```python
from build123d import *

# Parameters (mm, degrees)
BOSS_EXTRUDE1_DEPTH      = 6.2
SKETCH2_W                = 5.2
SKETCH2_H                = 28
CUT_EXTRUDE1_DEPTH       = 15.5
SKETCH3_R                = 1.45
BOSS_EXTRUDE2_DEPTH      = 1
DOME1_FACE_RADIUS        = 1.45
DOME1_HEIGHT             = 1.45
SKETCH4_W                = 4
SKETCH4_H                = 8.2
BOSS_EXTRUDE3_DEPTH      = 5
SKETCH5_W                = 3
SKETCH5_H                = 3.5
CUT_EXTRUDE2_DEPTH       = 4.8
SKETCH6_W                = 4
SKETCH6_H                = 2
BOSS_EXTRUDE4_DEPTH      = 1.5
BOSS_EXTRUDE4_TAPER      = 15
BOSS_EXTRUDE5_DEPTH      = 3
BOSS_EXTRUDE5_DEPTH_BACK = 3
SKETCH8_R                = 2
CUT_EXTRUDE3_DEPTH       = 1.5
SKETCH9_R                = 2
CUT_EXTRUDE4_DEPTH       = 1.5
SKETCH10_R               = 2
CUT_EXTRUDE5_DEPTH       = 1.5
SKETCH11_W               = 5.2
SKETCH11_H               = 5.2
CUT_EXTRUDE6_DEPTH       = 2.5
CUT_EXTRUDE6_DRAFT       = -15
SKETCH12_W               = 5.2
SKETCH12_H               = 5.2
CUT_EXTRUDE7_DEPTH       = 2.5
CUT_EXTRUDE7_DRAFT       = -15
SKETCH13_W               = 5.2
SKETCH13_H               = 5.2
CUT_EXTRUDE8_DEPTH       = 2.5
CUT_EXTRUDE8_DRAFT       = -15
SKETCH14_W               = 5.2
SKETCH14_H               = 5.2
CUT_EXTRUDE9_DEPTH       = 2.5
CUT_EXTRUDE9_DRAFT       = -15
SKETCH15_W               = 5.2
SKETCH15_H               = 5.2
CUT_EXTRUDE10_DEPTH      = 2.5
CUT_EXTRUDE10_DRAFT      = -15


with BuildPart() as part:
    # Sketch1 → Boss-Extrude1 (new body)
    with BuildSketch(Plane(origin=(0, 0, 0), x_dir=(0, 0, -1), z_dir=(1, 0, 0))):
        Polygon((0, 0), (0, 3.5), (35, 3.5), (35, 2), (33.5, 2), (33.5, 0), (63.5, 0), (63.5, 16.5), (52, 16.5), (47.468461065, 14.386908691), (46.20060628, 17.105832052), (48.919529641, 18.373686838), (48.919529641, 19.8), (53.5, 19.8), (53.5, 35.663086876), (41.594285018, 35.663086876), (37.062746083, 33.549995567), (35.794891298, 36.268918928), (38.513814659, 37.536773714), (38.513814659, 38.963086876), (43.094285018, 38.963086876), (43.094285018, 55.2), (35.394285018, 55.2), (35.394285018, 68.074097914), (25.594285018, 70.7), (25.594285018, 55.2), (-0.105714982, 55.2), (-0.105714982, 70.7), (-8.705714982, 70.7), (-8.705714982, 55.2), (-16.405714982, 55.2), (-16.405714982, 38.963086876), (-11.825244622, 38.963086876), (-11.825244622, 37.536773714), (-9.106321261, 36.268918928), (-10.374176047, 33.549995567), (-14.905714982, 35.663086876), (-26.811429963, 35.663086876), (-26.811429963, 19.8), (-22.230959604, 19.8), (-22.230959604, 18.373686838), (-19.512036243, 17.105832052), (-20.779891028, 14.386908691), (-25.311429963, 16.5), (-26.811429963, 16.5), (-26.811429963, 11.5), (-18, 11.5), (-18, 0), align=None)
    extrude(amount=BOSS_EXTRUDE1_DEPTH)

    # Sketch2 → Cut-Extrude1 (cut)
    with BuildSketch(Plane(origin=(0, 70.7, 0), x_dir=(1, 0, 0), z_dir=(0, 1, 0))):
        with Locations((3.1, 12.744285018)):
            Rectangle(SKETCH2_W, SKETCH2_H)
    extrude(amount=-CUT_EXTRUDE1_DEPTH, mode=Mode.SUBTRACT)

    # Sketch3 → Boss-Extrude2 (add)
    with BuildSketch(Plane(origin=(0, 70.7, 0), x_dir=(1, 0, 0), z_dir=(0, 1, 0))):
        with Locations(Location((3.1, -5.255714982, 0), (0, 0, 90))):
            Circle(SKETCH3_R)
    extrude(amount=BOSS_EXTRUDE2_DEPTH)

    # Dome1: a dome of height H over a round flat face of radius A is a cap of a sphere of radius (A * A + H * H) / (2 * H)
    dome1_r = (DOME1_FACE_RADIUS * DOME1_FACE_RADIUS + DOME1_HEIGHT * DOME1_HEIGHT) / (2 * DOME1_HEIGHT)
    dome1_base = Plane((3.1, 71.7, 5.255714982), z_dir=(0, 1, 0))
    with Locations(dome1_base.offset(DOME1_HEIGHT - dome1_r)):
        dome1_ball = Sphere(dome1_r, mode=Mode.PRIVATE)
    add(split(dome1_ball, bisect_by=dome1_base, keep=Keep.TOP, mode=Mode.PRIVATE))

    # Sketch4 → Boss-Extrude3 (add)
    with BuildSketch(Plane.XY.offset(18)):
        with Locations((3.1, 4.3)):
            Rectangle(SKETCH4_W, SKETCH4_H)
    extrude(amount=BOSS_EXTRUDE3_DEPTH)

    # Sketch5 → Cut-Extrude2 (cut)
    with BuildSketch(Plane.XY.offset(23)):
        with Locations((3.6, 6.65)):
            Rectangle(SKETCH5_W, SKETCH5_H)
    extrude(amount=-CUT_EXTRUDE2_DEPTH, mode=Mode.SUBTRACT)

    # Sketch6 → Boss-Extrude4 (add)
    with BuildSketch(Plane(origin=(0, 0, 0), x_dir=(-1, 0, 0), z_dir=(0, 0, -1))):
        with Locations((-3.1, 1)):
            Rectangle(SKETCH6_W, SKETCH6_H)
    extrude(amount=BOSS_EXTRUDE4_DEPTH, taper=BOSS_EXTRUDE4_TAPER)

    # Sketch7 → Boss-Extrude5 (add, two sides: drawn at the far end of the back side and taken through both)
    with BuildSketch(Plane(origin=(3.1, 0, 0), x_dir=(0, 0, -1), z_dir=(1, 0, 0)).offset(-BOSS_EXTRUDE5_DEPTH_BACK)):
        Polygon((34.380497445, 68.345741476), (23.755313356, 71.192750972), (23.755313356, 73.792750972), (23.496494311, 74.758676798), (23.496494311, 76.692750972), (24.496494311, 76.692750972), (24.496494311, 75.692750972), (25.996494311, 75.692750972), (26.824715255, 72.601788328), (31.654344387, 71.307693102), (34.425625679, 72.907693102), (35.425625679, 72.907693102), (35.425625679, 68.907693102), align=None)
    extrude(amount=BOSS_EXTRUDE5_DEPTH + BOSS_EXTRUDE5_DEPTH_BACK)

    # Sketch8 → Cut-Extrude3 (cut)
    with BuildSketch(Plane(origin=(0, 55.2, 0), x_dir=(1, 0, 0), z_dir=(0, 1, 0))):
        with Locations(Location((3.1, 39.244285018, 0), (0, 0, 270))):
            Circle(SKETCH8_R)
        with Locations(Location((3.1, -12.555714982, 0), (0, 0, 270))):
            Circle(SKETCH8_R)
    extrude(amount=-CUT_EXTRUDE3_DEPTH, mode=Mode.SUBTRACT)

    # Sketch9 → Cut-Extrude4 (cut)
    with BuildSketch(Plane(origin=(0, 35.663086876, 0), x_dir=(1, 0, 0), z_dir=(0, 1, 0))):
        with Locations(Location((3.1, 47.547142509, 0), (0, 0, 270))):
            Circle(SKETCH9_R)
        with Locations(Location((3.1, -20.858572473, 0), (0, 0, 270))):
            Circle(SKETCH9_R)
    extrude(amount=-CUT_EXTRUDE4_DEPTH, mode=Mode.SUBTRACT)

    # Sketch10 → Cut-Extrude5 (cut)
    with BuildSketch(Plane(origin=(0, 16.5, 0), x_dir=(1, 0, 0), z_dir=(0, 1, 0))):
        with Locations(Location((3.1, 57.75, 0), (0, 0, 270))):
            Circle(SKETCH10_R)
    extrude(amount=-CUT_EXTRUDE5_DEPTH, mode=Mode.SUBTRACT)


with BuildPart() as cut_extrude6_tool:
    # Sketch11 → Cut-Extrude6 (with draft: the straight prism first)
    with BuildSketch(Plane(origin=(0, 0, -63.5), x_dir=(-1, 0, 0), z_dir=(0, 0, -1))):
        with Locations((-3.1, 5.6)):
            Rectangle(SKETCH11_W, SKETCH11_H)
    extrude(amount=-CUT_EXTRUDE6_DEPTH)
    # Cut-Extrude6: the draft: its side faces are tilted about the plane it starts from
    cut_extrude6_sides = [cut_extrude6_tool.faces().sort_by_distance(p)[0] for p in [
        (3.1, 3, -62.25),
        (0.5, 5.6, -62.25),
        (3.1, 8.2, -62.25),
        (5.7, 5.6, -62.25),
    ]]
    draft(cut_extrude6_sides, Plane(origin=(0, 0, -63.5), x_dir=(-1, 0, 0), z_dir=(0, 0, -1)), CUT_EXTRUDE6_DRAFT)


with BuildPart() as part_1:
    add(part.part)

    # Cut-Extrude6: cut by cut_extrude6_tool
    add(cut_extrude6_tool.part, mode=Mode.SUBTRACT)


with BuildPart() as cut_extrude7_tool:
    # Sketch12 → Cut-Extrude7 (with draft: the straight prism first)
    with BuildSketch(Plane(origin=(0, 0, -53.5), x_dir=(-1, 0, 0), z_dir=(0, 0, -1))):
        with Locations((-3.1, 25.4)):
            Rectangle(SKETCH12_W, SKETCH12_H)
    extrude(amount=-CUT_EXTRUDE7_DEPTH)
    # Cut-Extrude7: the draft: its side faces are tilted about the plane it starts from
    cut_extrude7_sides = [cut_extrude7_tool.faces().sort_by_distance(p)[0] for p in [
        (3.1, 22.8, -52.25),
        (0.5, 25.4, -52.25),
        (3.1, 28, -52.25),
        (5.7, 25.4, -52.25),
    ]]
    draft(cut_extrude7_sides, Plane(origin=(0, 0, -53.5), x_dir=(-1, 0, 0), z_dir=(0, 0, -1)), CUT_EXTRUDE7_DRAFT)


with BuildPart() as part_2:
    add(part_1.part)

    # Cut-Extrude7: cut by cut_extrude7_tool
    add(cut_extrude7_tool.part, mode=Mode.SUBTRACT)


with BuildPart() as cut_extrude8_tool:
    # Sketch13 → Cut-Extrude8 (with draft: the straight prism first)
    with BuildSketch(Plane(origin=(0, 0, -43.094285018), x_dir=(-1, 0, 0), z_dir=(0, 0, -1))):
        with Locations((-3.1, 44.563086876)):
            Rectangle(SKETCH13_W, SKETCH13_H)
    extrude(amount=-CUT_EXTRUDE8_DEPTH)
    # Cut-Extrude8: the draft: its side faces are tilted about the plane it starts from
    cut_extrude8_sides = [cut_extrude8_tool.faces().sort_by_distance(p)[0] for p in [
        (3.1, 41.963086876, -41.844285018),
        (0.5, 44.563086876, -41.844285018),
        (3.1, 47.163086876, -41.844285018),
        (5.7, 44.563086876, -41.844285018),
    ]]
    draft(cut_extrude8_sides, Plane(origin=(0, 0, -43.094285018), x_dir=(-1, 0, 0), z_dir=(0, 0, -1)), CUT_EXTRUDE8_DRAFT)


with BuildPart() as part_3:
    add(part_2.part)

    # Cut-Extrude8: cut by cut_extrude8_tool
    add(cut_extrude8_tool.part, mode=Mode.SUBTRACT)


with BuildPart() as cut_extrude9_tool:
    # Sketch14 → Cut-Extrude9 (with draft: the straight prism first)
    with BuildSketch(Plane.XY.offset(26.811429963)):
        with Locations((3.1, 25.4)):
            Rectangle(SKETCH14_W, SKETCH14_H)
    extrude(amount=-CUT_EXTRUDE9_DEPTH)
    # Cut-Extrude9: the draft: its side faces are tilted about the plane it starts from
    cut_extrude9_sides = [cut_extrude9_tool.faces().sort_by_distance(p)[0] for p in [
        (3.1, 22.8, 25.561429963),
        (5.7, 25.4, 25.561429963),
        (3.1, 28, 25.561429963),
        (0.5, 25.4, 25.561429963),
    ]]
    draft(cut_extrude9_sides, Plane.XY.offset(26.811429963), CUT_EXTRUDE9_DRAFT)


with BuildPart() as part_4:
    add(part_3.part)

    # Cut-Extrude9: cut by cut_extrude9_tool
    add(cut_extrude9_tool.part, mode=Mode.SUBTRACT)


with BuildPart() as cut_extrude10_tool:
    # Sketch15 → Cut-Extrude10 (with draft: the straight prism first)
    with BuildSketch(Plane.XY.offset(16.405714982)):
        with Locations((3.1, 44.563086876)):
            Rectangle(SKETCH15_W, SKETCH15_H)
    extrude(amount=-CUT_EXTRUDE10_DEPTH)
    # Cut-Extrude10: the draft: its side faces are tilted about the plane it starts from
    cut_extrude10_sides = [cut_extrude10_tool.faces().sort_by_distance(p)[0] for p in [
        (3.1, 41.963086876, 15.155714982),
        (5.7, 44.563086876, 15.155714982),
        (3.1, 47.163086876, 15.155714982),
        (0.5, 44.563086876, 15.155714982),
    ]]
    draft(cut_extrude10_sides, Plane.XY.offset(16.405714982), CUT_EXTRUDE10_DRAFT)


with BuildPart() as part_5:
    add(part_4.part)

    # Cut-Extrude10: cut by cut_extrude10_tool
    add(cut_extrude10_tool.part, mode=Mode.SUBTRACT)


solid = part_5.part
```
Read the model definition and answer for the solid it produces. Units are mm, in the model's axes. A direction names the side the tool comes from. Coordinates: 2 decimals unless noted, no trailing zeros. Loops run counter-clockwise (first coordinate to the right, second up) from the corner with the lowest first, then second, coordinate; pieces in that order, holes last.
(1) The mould has two halves that part along Z. Classify faces 1 (the face through (3.14, 3.33, -62.27)), 2 (the face through (3.064, 42.293, 15.173)), 3 (the face through (6.2, 28, -18)), 4 (the face through (3.06, 15.46, -49.77)): released by +Z, released by -Z, zero draft, split by the parting line, or undercut.
Solution:
face 1: released by -Z
face 2: released by +Z
face 3: zero draft
face 4: undercut
(2) The part is cut by section C-C (y = 51.5). Determine the outline of the cut face in (x, z), and give its area (3 significant figures).
Solution:
outline: (0, -43.09) - (6.2, -43.09) - (6.2, 16.41) - (0, 16.41) - close
area: 369 mm2
(3) A tool of negligible diameter and unlimited length cuts with its end or side. For faces 5 (the face through (3.06, 34.89, -36.44)), 6 (the face through (3, 49, -43.094)), 7 (the face through (5.37, 44.53, 15.17)), 8 (the face through (1.9, 8.4, 20.3)), from which of +Z, -Z, +X, -X, +Y, -Y can it reach the whole face along a straight path? Write none if from no direction.
Solution:
face 5: +X, -X
face 6: -Z, +X, -X, +Y
face 7: +Z
face 8: +Z, +X, -X
(4) Flat-ended cylindrical pins translate along their axes: pin 1 Ø2 at (x, y) = (3.5, 75.5) entering from +Z; pin 2 Ø3.5 at (x, z) = (3.1, -57.75) entering from -Y; pin 3 Ø2.5 at (y, z) = (4, 20.5) entering from +X; pin 4 Ø2 at (x, z) = (2, 20.5) entering from +Y. Find the tip coordinate at first contact, or state that the pin passes through.
Solution:
pin 1: stops at z = -23.5
pin 2: stops at y = 0
pin 3: stops at x = 5.1
pin 4: stops at y = 35.66
(5) The part is cut by section A-A (z = -57.75). Determine the outline of the cut face in (x, y), and give its area (3 significant figures).
Solution:
outline: (0, 0) - (6.2, 0) - (6.2, 16.5) - (5.1, 16.5) - (5.1, 15) - (1.1, 15) - (1.1, 16.5) - (0, 16.5) - close
area: 96.3 mm2
(6) The part is cut by section B-B (y = 26). Determine the outline of the cut face in (x, z), and give its area (3 significant figures).
Solution:
outline: (0, -53.5) - (0.5, -53.5) - (1.17, -51) - (5.03, -51) - (5.7, -53.5) - (6.2, -53.5) - (6.2, 26.81) - (5.7, 26.81) - (5.03, 24.31) - (1.17, 24.31) - (0.5, 26.81) - (0, 26.81) - close
area: 475 mm2
(7) Consider line 1 along X through (y, z) = (70.5, 0.5); line 2 along Z through (x, y) = (1.75, 21); line 3 along Y through (x, z) = (3.5, 12). Determine where each line is inside the solid, lowest interval first.
Solution:
line 1: x = 0 to 0.5, 5.7 to 6.2
line 2: z = -53.5 to 26.81
line 3: y = 0 to 34.31, 38.96 to 53.7
